Design review of the part shown in the three views and the two pictorial views. Dimensions are in mm from the part's minimum x, y and z. A direction names the side the tool comes from. Round coordinates to 2 decimals unless told otherwise and drop trailing zeros. Loops run counter-clockwise (first coordinate to the right, second up) from the corner with the lowest first, then second, coordinate; pieces in that order, holes last.
1. Consider section A-A on x = 15. State the section outline as (y, z) points, then the cut area to 3 significant figures.
2. Consider section B-B on z = 3.5. State the section outline as (x, y) points (3 decimals).
3. Consider section C-C on y = 13.75. State the section outline as (x, z) points, then the cut area to 3 significant figures.
4. To check wall thickness, follow line 1 along X through (y, z) = (1.1, 3.5) (3 decimals); line 2 along Y through (x, z) = (10.75, 5); line 3 along Z through (x, y) = (21.25, 1.5) (3 decimals). State the ranges of each line that lie inside material, in increasing order.
5. Clearance check with flat-ended pins moving along their axes: pin 1 Ø12 at (x, y) = (3, 14.5) entering from -Z; pin 2 Ø2 at (x, z) = (14, 4.5) entering from +Y. State where each tip first meets the part, or that it passes through.
6. Consider section D-D on x = 4. State the section outline as (y, z) points.
7. Draft analysis for pull direction X (two halves, no side actions). For the marked faces 3, 4 and 5, state which applies: released by +X, released by -X, zero draft, split by the parting line, or undercut.
8. Tool access review of the marked faces 1 and 2: name each direction out of +Z, -Z, +X, -X, +Y, -Y from which nothing blocks a thin tool from reaching the whole face with its end or side.
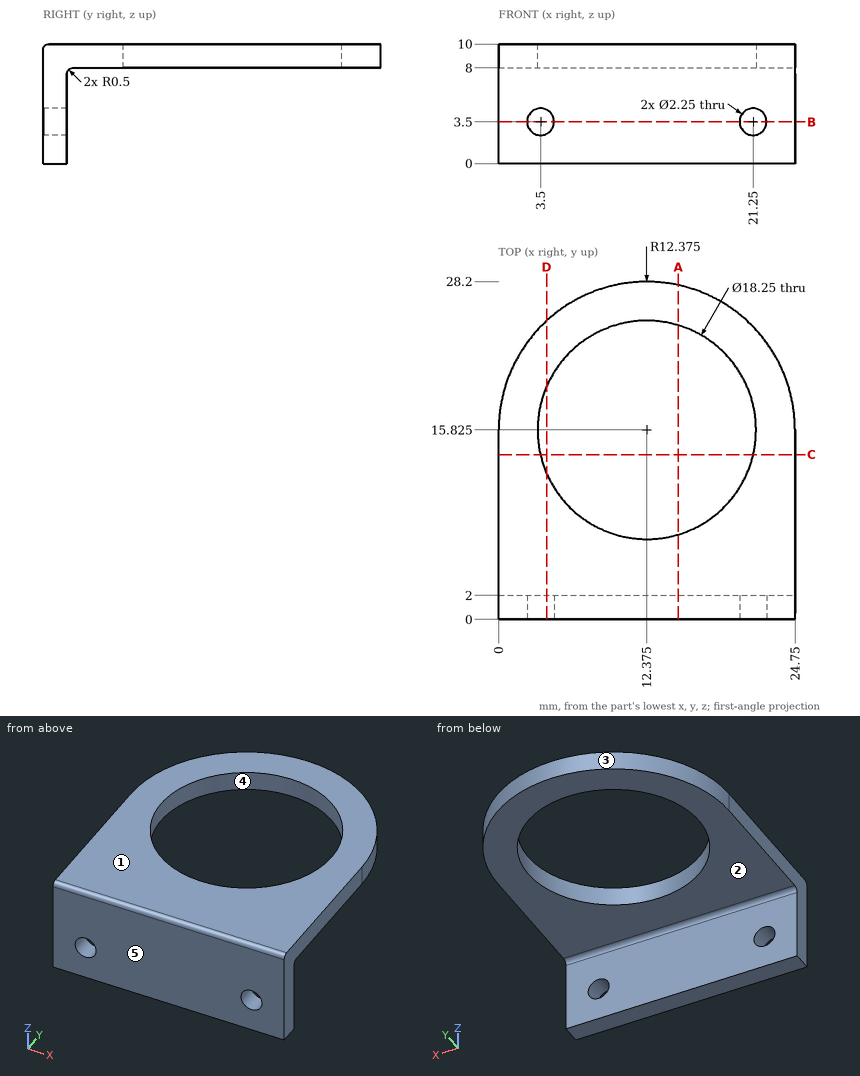
Resolved:
1. outline: (0, 0) - (2, 0) - (2, 7.5) arc R0.5 cw to (2.5, 8) - (7.09, 8) - (7.09, 10) - (0.5, 10) arc R0.5 ccw to (0, 9.5) - close; (24.56, 8) - (27.92, 8) - (27.92, 10) - (24.56, 10) - close
1. area: 36.9 mm2
2. outline: (0, 0) - (2.375, 0) - (2.375, 2) - (0, 2) - close; (4.625, 0) - (20.125, 0) - (20.125, 2) - (4.625, 2) - close; (22.375, 0) - (24.75, 0) - (24.75, 2) - (22.375, 2) - close
3. outline: (0, 8) - (3.49, 8) - (3.49, 10) - (0, 10) - close; (21.26, 8) - (24.75, 8) - (24.75, 10) - (21.26, 10) - close
3. area: 14.0 mm2
4. line 1: x = 0 to 2.375, 4.625 to 20.125, 22.375 to 24.75
4. line 2: y = 0 to 2
4. line 3: z = 0 to 2.375, 4.625 to 10
5. pin 1: stops at z = 8
5. pin 2: stops at y = 2
6. outline: (0, 0) - (2, 0) - (2, 2.49) - (0, 2.49) - close; (0, 4.51) - (2, 4.51) - (2, 7.5) arc R0.5 cw to (2.5, 8) - (12.2, 8) - (12.2, 10) - (0.5, 10) arc R0.5 ccw to (0, 9.5) - close; (19.45, 8) - (24.94, 8) - (24.94, 10) - (19.45, 10) - close
7. face 3: split by the parting line
7. face 4: undercut
7. face 5: zero draft
8. face 1: +Z, +X, -X, +Y, -Y
8. face 2: -Z, +X, -X, +Y
